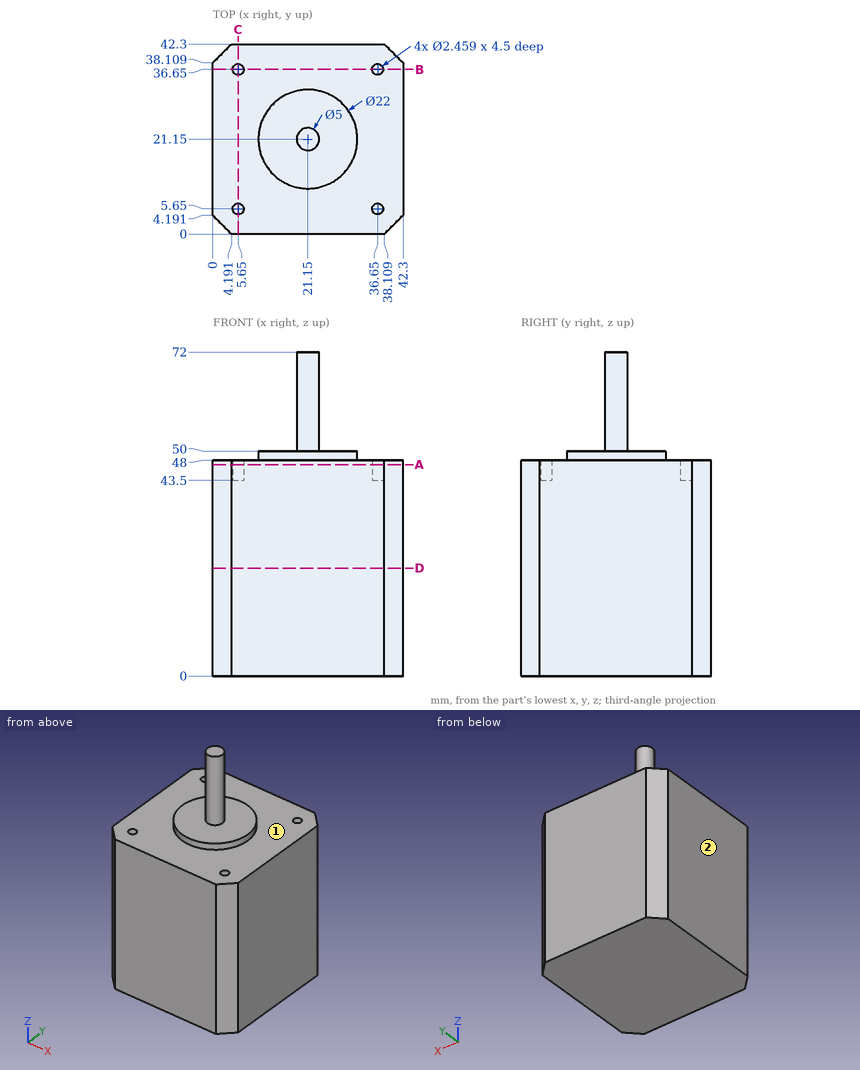
Can you work these out from the drawing? Everything is in mm from the part's minimum corner. A direction names the side the tool comes from. Give positions to 0.01 mm unless a question says otherwise; leave off trailing zeros. Order: outer loops, then holes, each group sorted by start corner. A loop starts at its lowest first (then second) coordinate and runs counter-clockwise, first axis right, second up. Notation, with made-up numbers: M 19.5,-20.75 L 40.5,-20.75 A26 cw 40.5,9.25 Z; hole C -8.75,44 d2. An arc over 180 degrees is marked long. Use a Markdown table: item, result. Add a question column.
Item 1: If I drill on L1, parallel to Y at x = 5.65, z = 47.05; L2, parallel to Y at x = 36, z = 46 (1 decimal), over which ranges is the centre line in solid material (lowest first)? Write a range as [from, to].
Item 2: Suppose I cut it at B-B (y = 36.65). List the corners of the cut face in (x, z) for me, then the cut area to 3 significant figures.
Item 3: Will these pins go through, and if not, where does the flat tip stop? pin 1 (0.7 mm diameter, centred on x = 37, y = 5.5, fed in from +Z); pin 2 (3 mm diameter, centred on x = 36.65, y = 36.65, fed in from +Z); pin 3 (2 mm diameter, centred on y = 20, z = 49.5, fed in from -X).
Item 4: For the marked faces 1 and 2, which set-ups out of +Z, -Z, +X, -X, +Y, -Y let a thin tool reach every point of the face, with its end or its side?
Item 5: Suppose I cut it at D-D (z = 24). List the corners of the cut face in (x, y) for me, then the cut area to 3 significant figures.
Item 6: Suppose I cut it at A-A (z = 47). List the corners of the cut face in (x, y) for me, then the cut area to 3 significant figures.
Answer sheet:
| question | item | result |
|---|---|---|
| 1 | L1 | y = [0, 4.42], [6.88, 35.42], [37.88, 42.3] |
| 1 | L2 | y = [0, 4.6], [6.7, 35.6], [37.7, 42.3] |
| 2 | outline | M 0,0 L 42.3,0 L 42.3,48 L 37.88,48 L 37.88,43.5 L 35.42,43.5 L 35.42,48 L 6.88,48 L 6.88,43.5 L 4.42,43.5 L 4.42,48 L 0,48 Z |
| 2 | area | 2,010 mm² |
| 3 | pin 1 | stops at z = 43.5 |
| 3 | pin 2 | stops at z = 48 |
| 3 | pin 3 | stops at x = 10.15 |
| 4 | face 1 | +Z |
| 4 | face 2 | +Z, -Z, -X, +Y, -Y |
| 5 | outline | M 0,4.19 L 4.19,0 L 38.11,0 L 42.3,4.19 L 42.3,38.11 L 38.11,42.3 L 4.19,42.3 L 0,38.11 Z |
| 5 | area | 1,750 mm² |
| 6 | outline | M 0,4.19 L 4.19,0 L 38.11,0 L 42.3,4.19 L 42.3,38.11 L 38.11,42.3 L 4.19,42.3 L 0,38.11 Z; hole C 5.65,5.65 d2.46; hole C 5.65,36.65 d2.46; hole C 36.65,5.65 d2.46; hole C 36.65,36.65 d2.46 |
| 6 | area | 1,740 mm² |
